Geometry check sheet. Reference: the model listing, model coordinates, mm. Face numbers are marked on the shaded views. A direction names the side the tool comes from. Coordinates: 2 decimals unless noted, no trailing zeros. Loops run counter-clockwise (first coordinate to the right, second up) from the corner with the lowest first, then second, coordinate; pieces in that order, holes last. Notation, with made-up numbers: (-17, 3) - (2, 3) arc R29 ccw to (2, 37) - close; hole circle Ø2 at (50, 46.5). An arc over 180 degrees is marked (long way). Write each question's results on one line, items separated by ' | '. Start each with the question number.
(1) Sectioned sample at B-B (y = -22.5). Enter the section's corners in (x, z), plus the area to 3 significant figures.
(2) Go/stop test with flat-tipped pins: pin 1 Ø14 at (x, z) = (15, -22) entering from +Y; pin 2 Ø9 at (x, y) = (8, -20) entering from +Z; pin 3 Ø12 at (x, y) = (12.5, -37.5) entering from +Z. Record where each tip stops, or that it passes through.
(3) Material ranges on probe 1 along Y at (x, z) = (1.75, -21); probe 2 along X at (y, z) = (4, -22); probe 3 along Y at (x, z) = (9, -49), recorded low to high.
(4) Sectioned sample at C-C (z = -37). Enter the section's corners in (x, y).
(5) Access from +Z, -Z, +X, -X, +Y, -Y to the whole of each face (thin tool, end or side, straight path). Record for the marked faces 4, 5 and 6.
(6) Sectioned sample at D-D (y = 4). Enter the section's corners in (x, z).
(7) Sectioned sample at A-A (x = 15). Enter the section's corners in (y, z), plus the area to 3 significant figures.
(8) Mould release check, pull along Y, two halves, no side actions. Record for the marked faces 1, 2 and 3: pulls with the +Y half, pulls with the -Y half, needs draft (parallel to the pull), parting line crosses it, or undercut.
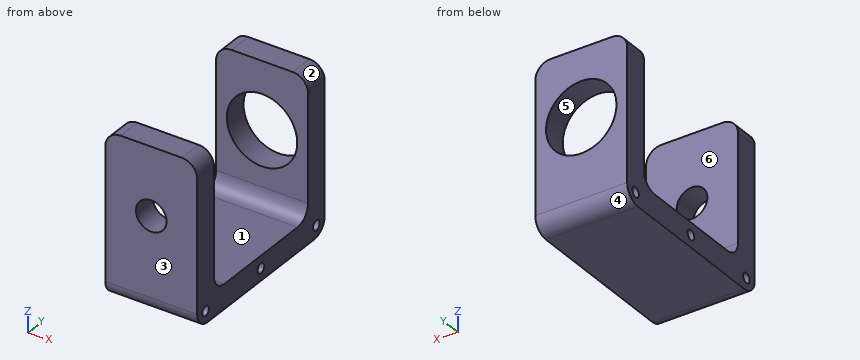
from build123d import *

# Parameters (mm, degrees)
BOSS_EXTRUDE1_DEPTH = 30
CUT_EXTRUDE1_REACH  = 88.197
SKETCH2_R           = 11.5
CUT_EXTRUDE2_REACH  = 82.734
SKETCH3_R           = 5
CUT_EXTRUDE3_REACH  = 82.734
SKETCH4_R           = 1.6
FILLET1_R           = 5
FILLET2_R           = 5


with BuildPart() as part:
    # Sketch1 → Boss-Extrude1 (new body)
    with BuildSketch(Plane(origin=(0, 0, 0), x_dir=(0, 0, -1), z_dir=(1, 0, 0))):
        Polygon((0, 0), (45, 0), (45, -45), (0, -45), (0, -53), (53, -53), (53, 8), (0, 8), align=None)
    extrude(amount=BOSS_EXTRUDE1_DEPTH)

    # Sketch2 → Cut-Extrude1 (cut, up to next)
    with BuildSketch(Plane(origin=(0, 8, 0), x_dir=(1, 0, 0), z_dir=(0, 1, 0)), mode=Mode.PRIVATE) as cut_extrude1_sk1:
        with Locations(Location((15, 22, 0), (0, 0, 270))):
            Circle(SKETCH2_R)
    cut_extrude1_tool1 = extrude(cut_extrude1_sk1.sketch, amount=-CUT_EXTRUDE1_REACH, mode=Mode.PRIVATE) & part.part
    add(cut_extrude1_tool1.solids().sort_by_distance((15, 8, -22))[0], mode=Mode.SUBTRACT)

    # Sketch3 → Cut-Extrude2 (cut, up to next)
    with BuildSketch(Plane(origin=(0, -45, 0), x_dir=(1, 0, 0), z_dir=(0, 1, 0)), mode=Mode.PRIVATE) as cut_extrude2_sk1:
        with Locations(Location((15, 22, 0), (0, 0, 270))):
            Circle(SKETCH3_R)
    cut_extrude2_tool1 = extrude(cut_extrude2_sk1.sketch, amount=-CUT_EXTRUDE2_REACH, mode=Mode.PRIVATE) & part.part
    add(cut_extrude2_tool1.solids().sort_by_distance((15, -45, -22))[0], mode=Mode.SUBTRACT)

    # Sketch4 → Cut-Extrude3 (cut, up to next)
    with BuildSketch(Plane(origin=(30, 0, 0), x_dir=(0, 0, -1), z_dir=(1, 0, 0)), mode=Mode.PRIVATE) as cut_extrude3_sk1:
        with Locations((49, -22.5)):
            Circle(SKETCH4_R)
    cut_extrude3_tool1 = extrude(cut_extrude3_sk1.sketch, amount=-CUT_EXTRUDE3_REACH, mode=Mode.PRIVATE) & part.part
    # Sketch4 → Cut-Extrude3 (cut, up to next)
    with BuildSketch(Plane(origin=(30, 0, 0), x_dir=(0, 0, -1), z_dir=(1, 0, 0)), mode=Mode.PRIVATE) as cut_extrude3_sk2:
        with Locations((49, -49)):
            Circle(SKETCH4_R)
    cut_extrude3_tool2 = extrude(cut_extrude3_sk2.sketch, amount=-CUT_EXTRUDE3_REACH, mode=Mode.PRIVATE) & part.part
    # Sketch4 → Cut-Extrude3 (cut, up to next)
    with BuildSketch(Plane(origin=(30, 0, 0), x_dir=(0, 0, -1), z_dir=(1, 0, 0)), mode=Mode.PRIVATE) as cut_extrude3_sk3:
        with Locations((49, 4)):
            Circle(SKETCH4_R)
    cut_extrude3_tool3 = extrude(cut_extrude3_sk3.sketch, amount=-CUT_EXTRUDE3_REACH, mode=Mode.PRIVATE) & part.part
    add(cut_extrude3_tool1.solids().sort_by_distance((30, -22.5, -49))[0], mode=Mode.SUBTRACT)
    add(cut_extrude3_tool2.solids().sort_by_distance((30, -49, -49))[0], mode=Mode.SUBTRACT)
    add(cut_extrude3_tool3.solids().sort_by_distance((30, 4, -49))[0], mode=Mode.SUBTRACT)

    # Fillet1
    fillet1_edges = [part.edges().sort_by_distance(p)[0] for p in [
        (0, 4, 0),
        (15, 8, -53),
        (15, -53, -53),
        (30, -49, 0),
        (30, 4, 0),
        (0, -49, 0),
    ]]
    fillet(fillet1_edges, radius=FILLET1_R)

    # Fillet2
    fillet2_edges = [part.edges().sort_by_distance(p)[0] for p in [
        (15, -45, -45),
        (15, 0, -45),
    ]]
    fillet(fillet2_edges, radius=FILLET2_R)


solid = part.part
Outcome:
1) outline: (0, -53) - (30, -53) - (30, -50.6) - (0, -50.6) - close; (0, -47.4) - (30, -47.4) - (30, -45) - (0, -45) - close | area: 144 mm2
2) pin 1: stops at y = -45 | pin 2: stops at z = -45 | pin 3: stops at z = -43.57
3) probe 1: y = -53 to -45, 0 to 8 | probe 2: x = 0 to 3.5, 26.5 to 30 | probe 3: y = -52.9 to -50.6, -47.4 to -24.1, -20.9 to 2.4, 5.6 to 7.9
4) outline: (0, -53) - (30, -53) - (30, -45) - (0, -45) - close; (0, 0) - (30, 0) - (30, 8) - (0, 8) - close
5) face 4: -Z, +X, -X, +Y | face 5: +Y | face 6: +Z, +X, -X
6) outline: (0, -52.9) - (30, -52.9) - (30, -50.6) - (0, -50.6) - close; (0, -47.4) - (30, -47.4) - (30, -5) arc R5 ccw to (25, 0) - (5, 0) arc R5 ccw to (0, -5) - close; hole circle Ø23 at (15, -22)
7) outline: (-53, -48) arc R5 ccw to (-48, -53) - (3, -53) arc R5 ccw to (8, -48) - (8, -33.5) - (0, -33.5) - (0, -40) arc R5 cw to (-5, -45) - (-40, -45) arc R5 cw to (-45, -40) - (-45, -27) - (-53, -27) - close; (-53, -17) - (-45, -17) - (-45, 0) - (-53, 0) - close; (0, -10.5) - (8, -10.5) - (8, 0) - (0, 0) - close; hole circle Ø3.2 at (-49, -49); hole circle Ø3.2 at (-22.5, -49); hole circle Ø3.2 at (4, -49) | area: 920 mm2
8) face 1: undercut | face 2: needs draft | face 3: pulls with the -Y half
